For this review, take the finished solid that the model builds, in its own axes (mm). Coordinates: 2 decimals unless noted, no trailing zeros. Write each loop counter-clockwise with the first axis right and the second up, starting at its lowest first coordinate (ties: lowest second). Pieces come first, ordered by that corner, then holes. Notation, with made-up numbers: (10.25, -2.5) - (15.25, -2.5) arc R10 ccw to (15.25, 8.5) - close; hole circle Ø1 at (86, 35.25). An arc over 180 degrees is marked (long way). Use one line per item in the form item = value. Start each with the question number.
1) We need section B-B (y = -25). Give the boundary of the cut face in (x, z), plus the area to 3 significant figures.
2) We need section A-A (y = 0). Give the boundary of the cut face in (x, z), plus the area to 3 significant figures.
3) Insertion check: P1, Ø1, axis at y = -1, z = 0, coming from the +X side; P2, Ø1, axis at x = -13.5, z = 0.5, coming from the -Y side. Each pin has a flat end and moves straight along its axis. Give the tip position at first contact, or say it passes through.
4) For L1, parallel to Y at x = -25, z = 0.5; L2, parallel to Y at x = 0, z = 1.1; L3, parallel to X at y = 8, z = 1.05, list the stretches that pass through material, from the lowest coordinate up. Write a range as from..to.
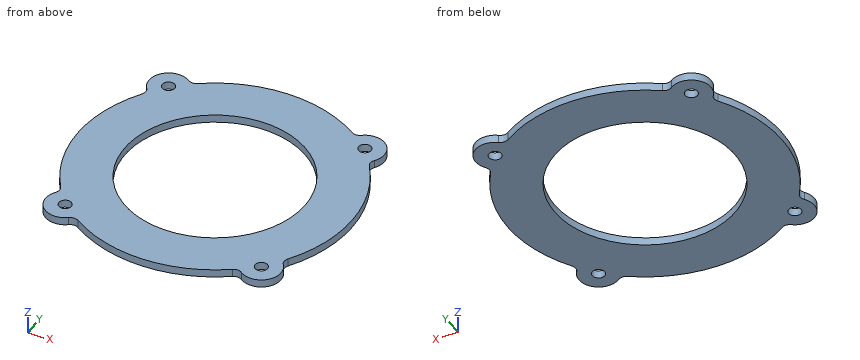
```python
from build123d import *

# Parameters (mm, degrees)
SKETCH1_R           = 23
SKETCH1_R_2         = 1.6
BOSS_EXTRUDE1_DEPTH = 2


with BuildPart() as part:
    # Sketch1 → Boss-Extrude1 (new body)
    with BuildSketch(Plane.XY):
        with BuildLine():
            ThreePointArc((-28.945945946, 19.675675676), (-35, 0), (-28.945945946, -19.675675676))
            ThreePointArc((-28.945945946, -19.675675676), (-28.600540614, -20.846499055), (-29, -22))
            ThreePointArc((-29, -22), (-28.535533906, -28.535533906), (-22, -29))
            ThreePointArc((-22, -29), (-20.846499055, -28.600540614), (-19.675675676, -28.945945946))
            ThreePointArc((-19.675675676, -28.945945946), (0, -35), (19.675675676, -28.945945946))
            ThreePointArc((19.675675676, -28.945945946), (20.846499055, -28.600540614), (22, -29))
            ThreePointArc((22, -29), (28.535533906, -28.535533906), (29, -22))
            ThreePointArc((29, -22), (28.600540614, -20.846499055), (28.945945946, -19.675675676))
            ThreePointArc((28.945945946, -19.675675676), (35, 0), (28.945945946, 19.675675676))
            ThreePointArc((28.945945946, 19.675675676), (28.600540614, 20.846499055), (29, 22))
            ThreePointArc((29, 22), (28.535533906, 28.535533906), (22, 29))
            ThreePointArc((22, 29), (20.846499055, 28.600540614), (19.675675676, 28.945945946))
            ThreePointArc((19.675675676, 28.945945946), (0, 35), (-19.675675676, 28.945945946))
            ThreePointArc((-19.675675676, 28.945945946), (-20.846499055, 28.600540614), (-22, 29))
            ThreePointArc((-22, 29), (-28.535533906, 28.535533906), (-29, 22))
            ThreePointArc((-29, 22), (-28.600540614, 20.846499055), (-28.945945946, 19.675675676))
        make_face()
        Circle(SKETCH1_R, mode=Mode.SUBTRACT)
        with Locations((-25, 25)):
            Circle(SKETCH1_R_2, mode=Mode.SUBTRACT)
        with Locations((25, 25)):
            Circle(SKETCH1_R_2, mode=Mode.SUBTRACT)
        with Locations((-25, -25)):
            Circle(SKETCH1_R_2, mode=Mode.SUBTRACT)
        with Locations((25, -25)):
            Circle(SKETCH1_R_2, mode=Mode.SUBTRACT)
    extrude(amount=BOSS_EXTRUDE1_DEPTH)


solid = part.part
```
Determined:
q1.outline = (-30, 0) - (-26.6, 0) - (-26.6, 2) - (-30, 2) - close; (-23.4, 0) - (23.4, 0) - (23.4, 2) - (-23.4, 2) - close; (26.6, 0) - (30, 0) - (30, 2) - (26.6, 2) - close
q1.area = 107 mm²
q2.outline = (-35, 0) - (-23, 0) - (-23, 2) - (-35, 2) - close; (23, 0) - (35, 0) - (35, 2) - (23, 2) - close
q2.area = 48.0 mm²
q3.P1 = 35
q3.P2 = -32.5
q4.L1 = -30..-26.6, -23.4..23.4, 26.6..30
q4.L2 = -35..-23, 23..35
q4.L3 = -34.07..-21.56, 21.56..34.07
